from build123d import *

# Parameters (mm, degrees)
BOSS_EXTRUDE1_DEPTH            = 77
SKETCH3_W                      = 37.54
SKETCH3_H                      = 17.27
BOSS_EXTRUDE2_DEPTH            = 1.77
SKETCH4_W                      = 37.54
SKETCH4_H                      = 17.27
BOSS_EXTRUDE3_DEPTH            = 1.77
SKETCH5_W                      = 4
SKETCH5_H                      = 16
CUT_EXTRUDE2_DEPTH             = 1.77
SKETCH6_W                      = 9.78
SKETCH6_H                      = 11.05
SKETCH6_W_2                    = 7.24
SKETCH6_H_2                    = 7.24
BUTTON_WALLS_DEPTH             = 7.24
SKETCH7_W                      = 9.78
SKETCH7_H                      = 11.05
BUTTON_BOTTOM_DEPTH            = 1.27
SKETCH8_W                      = 7.24
SKETCH8_H                      = 1.77
BUTTON_CUTOUT_MIDDLE_DEPTH     = 7.24
SKETCH9_W                      = 4.45
SKETCH9_H                      = 1.27
SKETCH9_W_2                    = 3.37
SKETCH9_H_2                    = 4.39
BUTTON_CUTOUT_FRONT_BACK_DEPTH = 7.24
SKETCH10_W                     = 3.37
SKETCH10_H                     = 4.39
BUTTON_CUTOUT_BOTTOM_DEPTH     = 1.27
BUTTON_CHAMFER1_SIZE           = 5
SKETCH12_W                     = 35
SKETCH12_H                     = 1.77
SKETCH12_W_2                   = 1.77
SKETCH12_H_2                   = 10
SKETCH12_W_3                   = 7.5
SKETCH12_R                     = 0.9652
SKETCH12_H_3                   = 7
SUPPORT_PCB_BATTERY_DEPTH      = 7
SKETCH13_W                     = 12
SKETCH13_H                     = 9
CUTOUT_USB_DEPTH               = 5
SKETCH14_W                     = 12.076722978
SKETCH14_H                     = 3.837896345
CUTOUT_TEMPORARY_DEPTH         = 5
SKETCH16_W                     = 1.77
SKETCH16_H                     = 1.77
TAB_PCB_RETAINER_DEPTH         = 3
SKETCH17_W                     = 4
SKETCH17_H                     = 1.77
CUTOUT_BACK_MOT_WIRES_DEPTH    = 9


with BuildPart() as part:
    # Sketch2 → Boss-Extrude1 (new body)
    with BuildSketch(Plane.XY):
        Polygon((-30.215355805, 3.088014981), (-30.215355805, -12.911985019), (4.784644195, -12.911985019), (4.784644195, 3.088014981), (6.054644195, 3.088014981), (6.054644195, -14.181985019), (-31.485355805, -14.181985019), (-31.485355805, 3.088014981), align=None)
    extrude(amount=BOSS_EXTRUDE1_DEPTH)

    # Sketch3 → Boss-Extrude2 (add)
    with BuildSketch(Plane.XY.offset(77)):
        with Locations((-12.715355805, -5.546985019)):
            Rectangle(SKETCH3_W, SKETCH3_H)
    extrude(amount=BOSS_EXTRUDE2_DEPTH)

    # Sketch4 → Boss-Extrude3 (add)
    with BuildSketch(Plane(origin=(0, 0, 0), x_dir=(-1, 0, 0), z_dir=(0, 0, -1))):
        with Locations((12.715355805, -5.546985019)):
            Rectangle(SKETCH4_W, SKETCH4_H)
    extrude(amount=BOSS_EXTRUDE3_DEPTH)

    # Sketch5 → Cut-Extrude2 (cut)
    with BuildSketch(Plane(origin=(0, 0, -1.77), x_dir=(-1, 0, 0), z_dir=(0, 0, -1))):
        with Locations((19.215355805, -4.911985019)):
            Rectangle(SKETCH5_W, SKETCH5_H)
    extrude(amount=-CUT_EXTRUDE2_DEPTH, mode=Mode.SUBTRACT)

    # Sketch6 → button_walls (add)
    with BuildSketch(Plane(origin=(0, 3.088014981, 0), x_dir=(1, 0, 0), z_dir=(0, 1, 0))):
        with Locations((-7.725355805, 1.135)):
            Rectangle(SKETCH6_W, SKETCH6_H)
        with Locations((-7.725355805, 1.77)):
            Rectangle(SKETCH6_W_2, SKETCH6_H_2, mode=Mode.SUBTRACT)
    extrude(amount=-BUTTON_WALLS_DEPTH)

    # Sketch7 → button_bottom (add)
    with BuildSketch(Plane.XZ.offset(4.151985019)):
        with Locations((-7.725355805, -1.135)):
            Rectangle(SKETCH7_W, SKETCH7_H)
    extrude(amount=BUTTON_BOTTOM_DEPTH)

    # Sketch8 → button_cutout_middle (cut)
    with BuildSketch(Plane(origin=(0, 3.088014981, 0), x_dir=(1, 0, 0), z_dir=(0, 1, 0))):
        with Locations((-7.725355805, 0.885)):
            Rectangle(SKETCH8_W, SKETCH8_H)
    extrude(amount=-BUTTON_CUTOUT_MIDDLE_DEPTH, mode=Mode.SUBTRACT)

    # Sketch9 → button_cutout_front_back (cut)
    with BuildSketch(Plane(origin=(0, 3.088014981, 0), x_dir=(1, 0, 0), z_dir=(0, 1, 0))):
        with Locations((-7.720355805, 6.025)):
            Rectangle(SKETCH9_W, SKETCH9_H)
        with Locations((-10.930355805, -2.195)):
            Rectangle(SKETCH9_W_2, SKETCH9_H_2)
        with Locations((-4.520355805, -2.195)):
            Rectangle(SKETCH9_W_2, SKETCH9_H_2)
    extrude(amount=-BUTTON_CUTOUT_FRONT_BACK_DEPTH, mode=Mode.SUBTRACT)

    # Sketch10 → button_cutout_bottom (cut)
    with BuildSketch(Plane(origin=(0, -4.151985019, 0), x_dir=(1, 0, 0), z_dir=(0, 1, 0))):
        with Locations((-10.930355805, -2.195)):
            Rectangle(SKETCH10_W, SKETCH10_H)
        with Locations((-4.520355805, -2.195)):
            Rectangle(SKETCH10_W, SKETCH10_H)
    extrude(amount=-BUTTON_CUTOUT_BOTTOM_DEPTH, mode=Mode.SUBTRACT)

    # button_Chamfer1
    # the kernel refuses this chamfer: 5 mm, written as the material it adds along each edge
    with BuildSketch(Plane(origin=(-6.205355805, -5.421985019, 0), x_dir=(0, -0.9996219169112968, -0.027495876610586372), z_dir=(-1, 0, 0))) as button_chamfer1_piece_1_section:
        Polygon((BUTTON_CHAMFER1_SIZE * 0.999621916911, BUTTON_CHAMFER1_SIZE * 0.0274958766106), (-BUTTON_CHAMFER1_SIZE * 0.0274958766106, BUTTON_CHAMFER1_SIZE * 0.999621916911), (0, 0), align=None)
    button_chamfer1_piece_1 = extrude(amount=3.04, mode=Mode.PRIVATE)
    button_chamfer1_piece_1 = split(button_chamfer1_piece_1, bisect_by=Plane(origin=(-7.725355805, -7.110612501, 4.39), z_dir=(0, 0, -1)), keep=Keep.TOP, mode=Mode.PRIVATE)
    add(button_chamfer1_piece_1)

    # Sketch12 → support_pcb_battery (add)
    # profile 1 of 5: a face of its own
    with BuildSketch(Plane(origin=(0, -12.911985019, 0), x_dir=(1, 0, 0), z_dir=(0, 1, 0))):
        with Locations((-12.715355805, -76.115)):
            Rectangle(SKETCH12_W, SKETCH12_H)
    # profile 2 of 5: a face of its own
    with BuildSketch(Plane(origin=(0, -12.911985019, 0), x_dir=(1, 0, 0), z_dir=(0, 1, 0))):
        with Locations((-27.100355805, -60.23)):
            Rectangle(SKETCH12_W_2, SKETCH12_H_2)
    # profile 3 of 5: a face of its own
    with BuildSketch(Plane(origin=(0, -12.911985019, 0), x_dir=(1, 0, 0), z_dir=(0, 1, 0))):
        with Locations((1.034644195, -36.845)):
            Rectangle(SKETCH12_W_3, SKETCH12_H)
    # profile 4 of 5: a face of its own
    with BuildSketch(Plane(origin=(0, -12.911985019, 0), x_dir=(1, 0, 0), z_dir=(0, 1, 0))):
        with BuildLine():
            Line((-25.783918863, -37.73), (-19.764792747, -37.73))
            ThreePointArc((-19.764792747, -37.73), (-22.774355805, -30.7466), (-25.783918863, -37.73))
        make_face()
        with Locations(Location((-22.774355805, -34.8868, 0), (0, 0, 270))):
            Circle(SKETCH12_R, mode=Mode.SUBTRACT)
    # profile 5 of 5: a face of its own
    with BuildSketch(Plane(origin=(0, -12.911985019, 0), x_dir=(1, 0, 0), z_dir=(0, 1, 0))):
        with Locations((-12.100355805, -23.33)):
            Rectangle(SKETCH12_W_2, SKETCH12_H_3)
    extrude(amount=SUPPORT_PCB_BATTERY_DEPTH)

    # Sketch13 → cutout_usb (cut)
    with BuildSketch(Plane(origin=(6.054644195, 0, 0), x_dir=(0, 0, -1), z_dir=(1, 0, 0))):
        with Locations((-24.395224713, -3.411985019)):
            Rectangle(SKETCH13_W, SKETCH13_H)
    extrude(amount=-CUTOUT_USB_DEPTH, mode=Mode.SUBTRACT)

    # Sketch14 → cutout_temporary (cut)
    with BuildSketch(Plane(origin=(6.054644195, 0, 0), x_dir=(0, 0, -1), z_dir=(1, 0, 0))):
        with Locations((-24.356863224, 3.006963154)):
            Rectangle(SKETCH14_W, SKETCH14_H)
    extrude(amount=-CUTOUT_TEMPORARY_DEPTH, mode=Mode.SUBTRACT)

    # Sketch16 → tab_pcb_retainer (add)
    with BuildSketch(Plane(origin=(0, -5.911985019, 0), x_dir=(1, 0, 0), z_dir=(0, 1, 0))):
        with Locations((-12.100355805, -20.715)):
            Rectangle(SKETCH16_W, SKETCH16_H)
    extrude(amount=TAB_PCB_RETAINER_DEPTH)

    # Sketch17 → cutout_back_mot_wires (cut)
    with BuildSketch(Plane(origin=(0, 3.088014981, 0), x_dir=(1, 0, 0), z_dir=(0, 1, 0))):
        with Locations((-20.361355805, -77.885)):
            Rectangle(SKETCH17_W, SKETCH17_H)
    extrude(amount=-CUTOUT_BACK_MOT_WIRES_DEPTH, mode=Mode.SUBTRACT)


solid = part.part
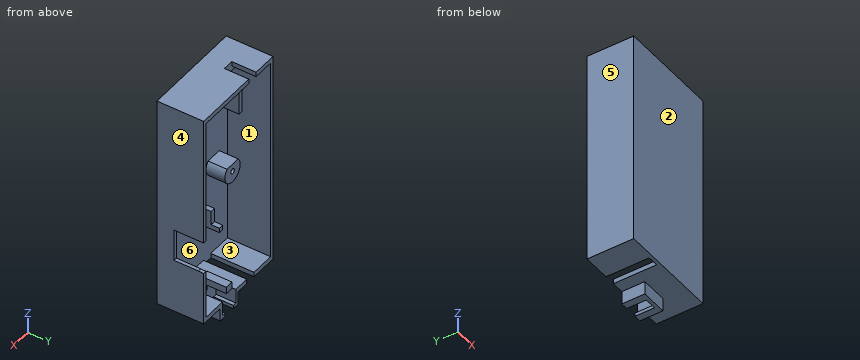
Model file for the job. Use its own axes, mm. Face numbers are marked on the shaded views. A direction names the side the tool comes from. Round coordinates to 2 decimals unless told otherwise and drop trailing zeros. Loops run counter-clockwise (first coordinate to the right, second up) from the corner with the lowest first, then second, coordinate; pieces in that order, holes last. Notation, with made-up numbers: (41.5, 55) -> (67.5, 55) arc R30 ccw to (67.5, 81) -> close; hole circle Ø3 at (19, 87.25). An arc over 180 degrees is marked (long way). Answer as CSV lines item,"result". Start each with the question number.
1) Tool access for the marked faces 1 and 2: list every direction of +Z, -Z, +X, -X, +Y, -Y with a clear straight run to the whole face (end or side of a thin tool).
2) Pin check, flat tips, straight feed: P1, Ø5, axis at x = -8, z = 32, coming from the +Y side; P2, Ø3, axis at x = -22.77, z = 34.89, coming from the +Y side; P3, Ø1.4, axis at x = -12.5, y = -9.5, coming from the -Z side; P4, Ø5, axis at y = -6.5, z = 24, coming from the +X side. Stop position of each tip, or through.
3) Mould opens along X. For the marked faces 3, 4, 5 and 6 say: +X half, -X half, draft (parallel to the pull), parting line (faces both ways), or undercut.
4) Slice it at A-A (z = 66). List the corners of the cut face in (x, y), plus the area to 3 significant figures.
5) Slice it at D-D (x = 2). List the corners of the cut face in (y, z).
6) Probe line 1 along Z through (x, y) = (-0.5, -8.5); line 2 along X through (y, z) = (-7.5, 2.5); line 3 along Z through (x, y) = (-26.5, 2.25). List the from-to ranges inside material, lowest first.
7) Slice it at B-B (y = -8.75). State how many separate pieces and enclosed holes the cut face has, plus the area to 3 significant figures.
Filled in:
1,face 1,"+Y"
1,face 2,"+Z, -Z, +X, -X, -Y"
2,P1,"stops at y = -12.91"
2,P2,"stops at y = -5.91"
2,P3,"stops at z = -1.77"
2,P4,"stops at x = 6.05"
3,face 3,"undercut"
3,face 4,"+X half"
3,face 5,"-X half"
3,face 6,"undercut"
4,outline,"(-31.49, -14.18) -> (6.05, -14.18) -> (6.05, 3.09) -> (4.78, 3.09) -> (4.78, -12.91) -> (-30.22, -12.91) -> (-30.22, 3.09) -> (-31.49, 3.09) -> close"
4,area,"88.3 mm2"
5,outline,"(-14.18, -1.77) -> (3.09, -1.77) -> (3.09, 0) -> (-12.91, 0) -> (-12.91, 35.96) -> (-5.91, 35.96) -> (-5.91, 37.73) -> (-12.91, 37.73) -> (-12.91, 75.23) -> (-5.91, 75.23) -> (-5.91, 77) -> (3.09, 77) -> (3.09, 78.77) -> (-14.18, 78.77) -> close"
6,line 1,"z = -1.77 to 0, 35.96 to 37.73, 75.23 to 78.77"
6,line 2,"x = -31.49 to -30.22, -9.25 to -6.21, 4.78 to 6.05"
6,line 3,"z = -1.77 to 0, 77 to 78.77"
7,separate pieces,"4"
7,enclosed holes,"1"
7,area,"477 mm2"
